from build123d import *

# Parameters (mm, degrees)
SKETCH1_R           = 10.5
BOSS_EXTRUDE2_DEPTH = 5


with BuildPart() as part:
    # Sketch1 → Boss-Extrude2 (new body)
    with BuildSketch(Plane(origin=(0, 0, 0), x_dir=(1, 0, 0), z_dir=(0, 1, 0))):
        with BuildLine():
            Line((16.516096513, -16.006828417), (52.2475067, 20.861400806))
            ThreePointArc((52.2475067, 20.861400806), (57.988295689, 29.675428199), (60, 40))
            ThreePointArc((60, 40), (42.426406871, 82.426406871), (0, 100))
            ThreePointArc((0, 100), (-42.426406871, 82.426406871), (-60, 40))
            ThreePointArc((-60, 40), (-57.988295689, 29.675428199), (-52.2475067, 20.861400806))
            Line((-52.2475067, 20.861400806), (-16.516096513, -16.006828417))
            ThreePointArc((-16.516096513, -16.006828417), (-8.967802028, -21.17967249), (0, -23))
            ThreePointArc((0, -23), (8.967802028, -21.17967249), (16.516096513, -16.006828417))
        make_face()
        with Locations(Location((32.5, 40, 0), (0, 0, 270))):
            Circle(SKETCH1_R, mode=Mode.SUBTRACT)
        with Locations(Location((-32.5, 40, 0), (0, 0, 90))):
            Circle(SKETCH1_R, mode=Mode.SUBTRACT)
        with BuildLine():
            Line((8.617093833, -8.351388739), (24.288887892, 7.819014071))
            ThreePointArc((24.288887892, 7.819014071), (28.192805121, 18.354250949), (23.055780503, 28.34638605))
            ThreePointArc((23.055780503, 28.34638605), (17.517341086, 40.721063014), (24.218531469, 52.506689369))
            ThreePointArc((24.218531469, 52.506689369), (32.255432897, 68.469423949), (22.572828784, 83.491003675))
            ThreePointArc((22.572828784, 83.491003675), (0, 89), (-22.572828784, 83.491003675))
            ThreePointArc((-22.572828784, 83.491003675), (-32.255432897, 68.469423949), (-24.218531469, 52.506689369))
            ThreePointArc((-24.218531469, 52.506689369), (-17.517341086, 40.721063014), (-23.055780503, 28.34638605))
            ThreePointArc((-23.055780503, 28.34638605), (-28.192805121, 18.354250949), (-24.288887892, 7.819014071))
            Line((-24.288887892, 7.819014071), (-8.617093833, -8.351388739))
            ThreePointArc((-8.617093833, -8.351388739), (-4.678853232, -11.050263908), (0, -12))
            ThreePointArc((0, -12), (4.678853232, -11.050263908), (8.617093833, -8.351388739))
        make_face(mode=Mode.SUBTRACT)
    extrude(amount=BOSS_EXTRUDE2_DEPTH)


solid = part.part
Source: CAD feature listing. Evaluate the final solid. Frame: model axes, mm. A direction names the side the tool comes from. Coordinates: 2 decimals unless noted, no trailing zeros. Loops run counter-clockwise (first coordinate to the right, second up) from the corner with the lowest first, then second, coordinate; pieces in that order, holes last. Notation, with made-up numbers: (23.25, 68.5) -> (32.25, 68.5) arc R20 cw to (32.25, 91.5) -> close; hole circle Ø10 at (-40, 57.25). An arc over 180 degrees is marked (long way). Answer in a Markdown table with one row per item. Add a question column.
Q1. Pull-direction query (Z, two-part tool) for faces 3 (the face through (-34.632, 2.465, -2.685)), 4 (the face through (-17.53, 2.46, -40.92)), 5 (the face through (26, 5, -53)); classes: pulls with the +Z half, pulls with the -Z half, needs draft (parallel to the pull), parting line crosses it, or undercut.
Q2. Contact query for flat-ended pins moving along their axis: pin 1 Ø12.5 at (x, z) = (-32.5, -40) entering from -Y; pin 2 Ø1 at (x, y) = (-26.5, 2) entering from -Z; pin 3 Ø3 at (x, y) = (26.5, 4) entering from -Z. Output: stop coordinate, or through.
Q3. Section B-B on z = -58. Return the cut outline in (x, y).
Q4. Section D-D on x = -30. Return the cut outline in (y, z), and give its area (3 significant figures).
Q5. Section C-C on x = 37. Return the cut outline in (y, z), and give its area (3 significant figures).
Q6. Ray query, line 1 along X through (y, z) = (2.85, -40); line 2 along X through (y, z) = (1.6, -49); line 3 along Z through (x, y) = (20, 3.1). Return the intervals inside material, ascending.
Q7. Section A-A on y = 2.7. Return the cut outline in (x, z), and give its area (3 significant figures).
Q8. Reachability of faces 1 (the face through (-16.563, 2.465, 0.153)), 2 (the face through (-58.044, 2.465, -29.813)) from +Z, -Z, +X, -X, +Y, -Y: full face, straight path, thin tool, end or side. Return the list, or none.
Computed values:
| question | item | result |
|---|---|---|
| 1 | face 3 | pulls with the +Z half |
| 1 | face 4 | undercut |
| 1 | face 5 | needs draft |
| 2 | pin 1 | passes through |
| 2 | pin 2 | stops at z = -94.07 |
| 2 | pin 3 | stops at z = -94.54 |
| 3 | outline | (-57.24, 0) -> (-29.56, 0) -> (-29.56, 5) -> (-57.24, 5) -> close; (29.56, 0) -> (57.24, 0) -> (57.24, 5) -> (29.56, 5) -> close |
| 4 | outline | (0, -91.96) -> (5, -91.96) -> (5, -76.28) -> (0, -76.28) -> close; (0, -58.75) -> (5, -58.75) -> (5, -50.2) -> (0, -50.2) -> close; (0, -29.8) -> (5, -29.8) -> (5, 2.09) -> (0, 2.09) -> close |
| 4 | area | 281 mm^2 |
| 5 | outline | (0, -87.23) -> (5, -87.23) -> (5, -49.49) -> (0, -49.49) -> close; (0, -30.51) -> (5, -30.51) -> (5, -5.13) -> (0, -5.13) -> close |
| 5 | area | 316 mm^2 |
| 6 | line 1 | x = -60 to -43, -22 to -17.5, 17.5 to 22, 43 to 60 |
| 6 | line 2 | x = -59.32 to -37.91, -27.09 to -20.5, 20.5 to 27.09, 37.91 to 59.32 |
| 6 | line 3 | z = -96.57 to -84.73, -48.29 to -31.71, -3.39 to 12.41 |
| 7 | outline | (-60, -40) arc R60 ccw to (60, -40) arc R27.5 ccw to (52.25, -20.86) -> (16.52, 16.01) arc R23 ccw to (-16.52, 16.01) -> (-52.25, -20.86) arc R27.5 ccw to start; hole circle Ø21 at (-32.5, -40); hole (-24.29, -7.82) arc R13.94 ccw to (-23.06, -28.35) arc R15 cw to (-24.22, -52.51) arc R18 ccw to (-22.57, -83.49) arc R49 ccw to (22.57, -83.49) arc R18 ccw to (24.22, -52.51) arc R15 cw to (23.06, -28.35) arc R13.94 ccw to (24.29, -7.82) -> (8.62, 8.35) arc R12 ccw to (-8.62, 8.35) -> close; hole circle Ø21 at (32.5, -40) |
| 7 | area | 5,240 mm^2 |
| 8 | face 1 | +Y, -Y |
| 8 | face 2 | +Z, -X, +Y, -Y |
